The model under review builds one solid part; all positions refer to its coordinate system, in mm. A direction names the side the tool comes from. Give positions to 0.01 mm unless a question says otherwise; leave off trailing zeros. Order: outer loops, then holes, each group sorted by start corner. A loop starts at its lowest first (then second) coordinate and runs counter-clockwise, first axis right, second up. Notation, with made-up numbers: (-26.75, 12.5) - (12.25, 12.5) arc R4 cw to (12.25, 18.5) - close; hole circle Ø11 at (8, 53.25). An arc over 180 degrees is marked (long way). Use a Markdown table: item, result. Add a question column.
```python
from build123d import *

# Parameters (mm, degrees)
SKETCH1_R           = 14.15
BOSS_EXTRUDE1_DEPTH = 3
SKETCH2_R           = 5
BOSS_EXTRUDE2_DEPTH = 21
SKETCH3_R           = 14.15
BOSS_EXTRUDE3_DEPTH = 3
SKETCH4_R           = 4
CUT_EXTRUDE1_DEPTH  = 34.607216487
CUT_EXTRUDE2_REACH  = 35.607
SKETCH5_R           = 1


with BuildPart() as part:
    # Sketch1 → Boss-Extrude1 (new body)
    with BuildSketch(Plane(origin=(0, 0, 0), x_dir=(1, 0, 0), z_dir=(0, 1, 0))):
        with Locations(Location((0, 0, 0), (0, 0, 270))):
            Circle(SKETCH1_R)
    extrude(amount=BOSS_EXTRUDE1_DEPTH)

    # Sketch2 → Boss-Extrude2 (add)
    with BuildSketch(Plane(origin=(0, 3, 0), x_dir=(1, 0, 0), z_dir=(0, 1, 0))):
        with Locations(Location((0, 0, 0), (0, 0, 90))):
            Circle(SKETCH2_R)
    extrude(amount=BOSS_EXTRUDE2_DEPTH)

    # Sketch3 → Boss-Extrude3 (add)
    with BuildSketch(Plane(origin=(0, 24, 0), x_dir=(1, 0, 0), z_dir=(0, 1, 0))):
        with Locations(Location((0, 0, 0), (0, 0, 270))):
            Circle(SKETCH3_R)
    extrude(amount=BOSS_EXTRUDE3_DEPTH)

    # Sketch4 → Cut-Extrude1 (cut, through all)
    with BuildSketch(Plane(origin=(0, 27, 0), x_dir=(1, 0, 0), z_dir=(0, 1, 0))):
        with Locations(Location((0, 0, 0), (0, 0, 270))):
            Circle(SKETCH4_R)
    extrude(amount=-CUT_EXTRUDE1_DEPTH, mode=Mode.SUBTRACT)

    # Sketch5 → Cut-Extrude2 (cut, up to next)
    with BuildSketch(Plane(origin=(0, 27, 0), x_dir=(1, 0, 0), z_dir=(0, 1, 0)), mode=Mode.PRIVATE) as cut_extrude2_sk1:
        with Locations(Location((-9, 0, 0), (0, 0, 270))):
            Circle(SKETCH5_R)
    cut_extrude2_tool1 = extrude(cut_extrude2_sk1.sketch, amount=-CUT_EXTRUDE2_REACH, mode=Mode.PRIVATE) & part.part
    # Sketch5 → Cut-Extrude2 (cut, up to next)
    with BuildSketch(Plane(origin=(0, 27, 0), x_dir=(1, 0, 0), z_dir=(0, 1, 0)), mode=Mode.PRIVATE) as cut_extrude2_sk2:
        with Locations(Location((-12.5, 0, 0), (0, 0, 270))):
            Circle(SKETCH5_R)
    cut_extrude2_tool2 = extrude(cut_extrude2_sk2.sketch, amount=-CUT_EXTRUDE2_REACH, mode=Mode.PRIVATE) & part.part
    add(cut_extrude2_tool1.solids().sort_by_distance((-9, 27, 0))[0], mode=Mode.SUBTRACT)
    add(cut_extrude2_tool2.solids().sort_by_distance((-12.5, 27, 0))[0], mode=Mode.SUBTRACT)


solid = part.part
```
Q1. We need section C-C (x = -12.5). Write out the cut boundary in (y, z), plus the area to 3 significant figures.
Q2. Clearance check with flat-ended pins moving along their axes: P1, Ø1.6, axis at x = -9, z = 0, coming from the +Y side; P2, Ø2, axis at y = 13.5, z = -1, coming from the -X side; P3, Ø8, axis at x = 4, y = 15.5, coming from the +Z side. State where each tip first meets the part, or that it passes through.
Q3. We need section D-D (z = -7.5). Write out the cut boundary in (x, y), plus the area to 3 significant figures.
Q4. We need section B-B (z = 0). Write out the cut boundary in (x, y), plus the area to 3 significant figures.
Q5. Wall thickness on probe 1 along X at (y, z) = (26.1, 0); probe 2 along Y at (x, z) = (3.25, -10.5); probe 3 along X at (y, z) = (15, 0): over which ranges is each line inside the solid? List them lowest first.
Q6. We need section A-A (x = 0). Write out the cut boundary in (y, z).
Q7. Machinability: for faces 1 (the flat face through (0, 24, 6)), 2 (the cylindrical face through (-5.42, 25.48, 13.07)), 3 (the cylindrical face through (-8, 26, 0)), which of the approach directions +Z, -Z, +X, -X, +Y, -Y give a long, thin tool a straight path to every point of the face, cutting with its end or side? Answer none if there is none.
Q8. Draft analysis for pull direction X (two halves, no side actions). For faces 4 (the cylindrical face through (-13.1, 25.5, -0.8)), 5 (the flat face through (-6, 3, 0)), 6 (the cylindrical face through (4.88, 13.35, 1.08)), state which applies: pulls with the +X half, pulls with the -X half, needs draft (parallel to the pull), parting line crosses it, or undercut.
Here are the results:
| question | item | result |
|---|---|---|
| 1 | outline | (0, -6.63) - (3, -6.63) - (3, 6.63) - (0, 6.63) - close; (24, -6.63) - (27, -6.63) - (27, -1) - (24, -1) - close; (24, 1) - (27, 1) - (27, 6.63) - (24, 6.63) - close |
| 1 | area | 73.6 mm2 |
| 2 | P1 | y = 3 |
| 2 | P2 | x = -5 |
| 2 | P3 | z = 5 |
| 3 | outline | (-12, 0) - (12, 0) - (12, 3) - (-12, 3) - close; (-12, 24) - (12, 24) - (12, 27) - (-12, 27) - close |
| 3 | area | 144 mm2 |
| 4 | outline | (-14.15, 0) - (-4, 0) - (-4, 27) - (-8, 27) - (-8, 24) - (-5, 24) - (-5, 3) - (-14.15, 3) - close; (-14.15, 24) - (-13.5, 24) - (-13.5, 27) - (-14.15, 27) - close; (-11.5, 24) - (-10, 24) - (-10, 27) - (-11.5, 27) - close; (4, 0) - (14.15, 0) - (14.15, 3) - (5, 3) - (5, 24) - (14.15, 24) - (14.15, 27) - (4, 27) - close |
| 4 | area | 152 mm2 |
| 5 | probe 1 | -14.15 to -13.5, -11.5 to -10, -8 to -4, 4 to 14.15 |
| 5 | probe 2 | 0 to 3, 24 to 27 |
| 5 | probe 3 | -5 to -4, 4 to 5 |
| 6 | outline | (0, -14.15) - (3, -14.15) - (3, -5) - (24, -5) - (24, -14.15) - (27, -14.15) - (27, -4) - (0, -4) - close; (0, 4) - (27, 4) - (27, 14.15) - (24, 14.15) - (24, 5) - (3, 5) - (3, 14.15) - (0, 14.15) - close |
| 7 | face 1 | none |
| 7 | face 2 | +Y, -Y |
| 7 | face 3 | +Y |
| 8 | face 4 | undercut |
| 8 | face 5 | needs draft |
| 8 | face 6 | parting line crosses it |
